from build123d import *

# Parameters (mm, degrees)
SKETCH1_W              = 25.4
SKETCH1_H              = 63.5
BASE_FLANGE1_DEPTH     = 1.7526
SKETCHED_BEND1_DEPTH   = 25.4
SKETCHED_BEND1_2_DEPTH = 25.4
CUT_EXTRUDE2_REACH     = 54.894
SKETCH9_R              = 3.302
SKETCH9_W              = 1.27
SKETCH9_H              = 5.08
SKETCH10_W             = 5.08
SKETCH10_H             = 5.08
BOSS_EXTRUDE1_DEPTH    = 1.7526
CUT_EXTRUDE3_REACH     = 54.894
SKETCH11_R             = 2.38125


# Read off the part's stored shape, not the designer's step: Sketched Bend1
# Sheet-metal steps are written as plain solids
with BuildPart() as part:
    # Sketch1 → Base-Flange1 (new body)
    with BuildSketch(Plane.XY):
        with Locations((12.7, 31.75)):
            Rectangle(SKETCH1_W, SKETCH1_H)
    extrude(amount=-BASE_FLANGE1_DEPTH)

    # Sketched Bend1 outline → Sketched Bend1 (cut)
    with BuildSketch(Plane.YZ):
        with BuildLine():
            Line((63.5, 0), (26.337912998, 0))
            ThreePointArc((26.337912998, 0), (25.005866723, -1.284495709), (23.215572088, -1.7526))
            Line((23.215572088, -1.7526), (63.5, -1.7526))
            Line((63.5, -1.7526), (63.5, 0))
        make_face()
    extrude(amount=SKETCHED_BEND1_DEPTH, mode=Mode.SUBTRACT)

    # Sketched Bend1 2 outline → Sketched Bend1 2 (add)
    with BuildSketch(Plane.YZ):
        with BuildLine():
            Line((25.120572088, 37.820572088), (25.120572088, 1.905))
            ThreePointArc((25.120572088, 1.905), (24.562610506, 0.557961582), (23.215572088, 0))
            Line((23.215572088, 0), (26.337912998, 0))
            ThreePointArc((26.337912998, 0), (26.736815609, 0.915615432), (26.873172088, 1.905))
            Line((26.873172088, 1.905), (26.873172088, 37.820572088))
            Line((26.873172088, 37.820572088), (25.120572088, 37.820572088))
        make_face()
    extrude(amount=SKETCHED_BEND1_2_DEPTH)

    # Sketch9 → Cut-Extrude2 (cut, up to next)
    with BuildSketch(Plane.XY, mode=Mode.PRIVATE) as cut_extrude2_sk1:
        with Locations((12.7, 12.7)):
            Circle(SKETCH9_R)
    cut_extrude2_tool1 = extrude(cut_extrude2_sk1.sketch, amount=-CUT_EXTRUDE2_REACH, mode=Mode.PRIVATE) & part.part
    # Sketch9 → Cut-Extrude2 (cut, up to next)
    with BuildSketch(Plane.XY, mode=Mode.PRIVATE) as cut_extrude2_sk2:
        with Locations((15.875, 2.54)):
            Rectangle(SKETCH9_W, SKETCH9_H)
    cut_extrude2_tool2 = extrude(cut_extrude2_sk2.sketch, amount=-CUT_EXTRUDE2_REACH, mode=Mode.PRIVATE) & part.part
    # Sketch9 → Cut-Extrude2 (cut, up to next)
    with BuildSketch(Plane.XY, mode=Mode.PRIVATE) as cut_extrude2_sk3:
        with Locations((9.525, 2.54)):
            Rectangle(SKETCH9_W, SKETCH9_H)
    cut_extrude2_tool3 = extrude(cut_extrude2_sk3.sketch, amount=-CUT_EXTRUDE2_REACH, mode=Mode.PRIVATE) & part.part
    add(cut_extrude2_tool1.solids().sort_by_distance((12.7, 12.7, 0))[0], mode=Mode.SUBTRACT)
    add(cut_extrude2_tool2.solids().sort_by_distance((15.875, 2.54, 0))[0], mode=Mode.SUBTRACT)
    add(cut_extrude2_tool3.solids().sort_by_distance((9.525, 2.54, 0))[0], mode=Mode.SUBTRACT)

    # Sketch10 → Boss-Extrude1 (add)
    with BuildSketch(Plane.XY):
        with Locations((-2.54, 12.7)):
            Rectangle(SKETCH10_W, SKETCH10_H)
    extrude(amount=-BOSS_EXTRUDE1_DEPTH)

    # Sketch11 → Cut-Extrude3 (cut, up to next)
    with BuildSketch(Plane(origin=(0, 26.873172088, 0), x_dir=(1, 0, 0), z_dir=(0, 1, 0)), mode=Mode.PRIVATE) as cut_extrude3_sk1:
        with Locations(Location((12.7, -25.154382, 0), (0, 0, 270))):
            Circle(SKETCH11_R)
    cut_extrude3_tool1 = extrude(cut_extrude3_sk1.sketch, amount=-CUT_EXTRUDE3_REACH, mode=Mode.PRIVATE) & part.part
    add(cut_extrude3_tool1.solids().sort_by_distance((12.7, 26.873172, 25.154382))[0], mode=Mode.SUBTRACT)


solid = part.part
Could you check a few things on this model? Use its own coordinates, in mm. A direction names the side the tool comes from. Give positions to 0.01 mm unless a question says otherwise; leave off trailing zeros. Order: outer loops, then holes, each group sorted by start corner. A loop starts at its lowest first (then second) coordinate and runs counter-clockwise, first axis right, second up. Notation, with made-up numbers: (1.25, -18.75) -> (32.25, -18.75) arc R13 ccw to (32.25, -6.75) -> close; hole circle Ø11 at (54, 9). An arc over 180 degrees is marked (long way). Return JSON: item names as keys, results as strings.
1. Imagine slicing it at C-C on z = 25. List the corners of the cut face in (x, y) for me, then the cut area to 3 significant figures.
Answer list:
{"outline": "(0, 25.12) -> (10.32, 25.12) -> (10.32, 26.87) -> (0, 26.87) -> close; (15.08, 25.12) -> (25.4, 25.12) -> (25.4, 26.87) -> (15.08, 26.87) -> close", "area": "36.2 mm2"}
2. Imagine slicing it at A-A on x = 12.7. List the corners of the cut face in (y, z) for me (3 decimals).
Answer list:
{"outline": "(0, -1.753) -> (9.398, -1.753) -> (9.398, 0) -> (0, 0) -> close; (16.002, -1.753) -> (23.216, -1.753) arc R3.658 ccw to (26.873, 1.905) -> (26.873, 22.773) -> (25.121, 22.773) -> (25.121, 1.905) arc R1.905 cw to (23.216, 0) -> (16.002, 0) -> close; (25.121, 27.536) -> (26.873, 27.536) -> (26.873, 37.821) -> (25.121, 37.821) -> close"}
3. Imagine slicing it at B-B on y = 4.25. List the corners of the cut face in (x, z) for me.
Answer list:
{"outline": "(0, -1.75) -> (8.89, -1.75) -> (8.89, 0) -> (0, 0) -> close; (10.16, -1.75) -> (15.24, -1.75) -> (15.24, 0) -> (10.16, 0) -> close; (16.51, -1.75) -> (25.4, -1.75) -> (25.4, 0) -> (16.51, 0) -> close"}
4. Imagine slicing it at D-D on y = 12.7. List the corners of the cut face in (x, z) for me, then the cut area to 3 significant figures.
Answer list:
{"outline": "(-5.08, -1.75) -> (9.4, -1.75) -> (9.4, 0) -> (-5.08, 0) -> close; (16, -1.75) -> (25.4, -1.75) -> (25.4, 0) -> (16, 0) -> close", "area": "41.8 mm2"}
5. Thinking about a two-plate mould opening in Y: for faces 5 (the cylindrical face through (12.27, 15.974, -0.864)), 6 (the flat face through (0, 5, -1)), 7 (the flat face through (10, 5.08, -1)), which applies, pulls with the +Y half, pulls with the -Y half, needs draft (parallel to the pull), parting line crosses it, or undercut?
Answer list:
{"face 5": "undercut", "face 6": "needs draft", "face 7": "pulls with the -Y half"}
6. For pin 1 Ø2 at (x, y) = (9.5, 7) entering from +Z; pin 2 Ø0.9 at (x, z) = (-3.5, -1) entering from +Y; pin 3 Ø1.4 at (y, z) = (1.5, -0.5) entering from -X, each with a flat end and sliding along its axis, tell me the tip position at first contact or that it passes through.
Answer list:
{"pin 1": "stops at z = 0", "pin 2": "stops at y = 15.24", "pin 3": "stops at x = 0"}
7. On a 3-axis mill with a long thin cutter (end or side, diameter ignored), from which of +Z, -Z, +X, -X, +Y, -Y can I reach the whole of each face in a straight line? I mean faces 1 (the flat face through (-3, 10.16, -1)), 2 (the flat face through (13, 25.121, 20)), 3 (the flat face through (0, 25.3, 15.2)), 4 (the flat face through (16, 5.08, -1)). Say none if no direction works.
Answer list:
{"face 1": "+Z, -Z, -X, -Y", "face 2": "+Z, +X, -X, -Y", "face 3": "+Z, -Z, -X, +Y", "face 4": "+Z, -Z, -Y"}
8. I need wall thicknesses on line 1 (Y direction, x = 18, z = 6.5); line 2 (Z direction, x = 9, y = 9); line 3 (Y direction, x = 12.7, z = -0.9). Which ranges of each line are inside material? Lowest first, please. Write a range as from..to.
Answer list:
{"line 1": "y = 25.12..26.87", "line 2": "z = -1.75..0", "line 3": "y = 0..9.4, 16..25.56"}
